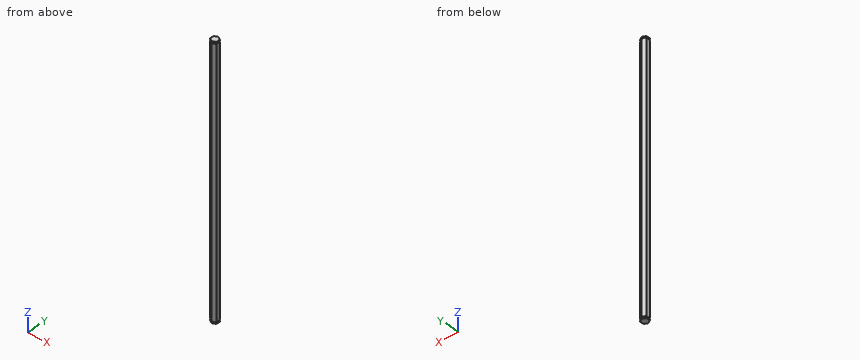
Solid Edge part; units mm, degrees
sketch "Sketch1" plane through (0, 0, 0) normal (0, 0, 1) x (1, 0, 0)
  line L0 (-6.1009, 4.0673) -> (-6.5728, -3.2499)
  line L1 (-6.5728, -3.2499) -> (-0.4719, -7.3171)
  line L2 (-0.4719, -7.3171) -> (6.1009, -4.0673)
  line L3 (6.1009, -4.0673) -> (6.5728, 3.2499)
  line L4 (6.5728, 3.2499) -> (0.4719, 7.3171)
  line L5 (0.4719, 7.3171) -> (-6.1009, 4.0673)
extrude "Protrusion1" add sketch "Sketch1" against normal blind 528.58
sketch "Sketch2" plane through (0, 0, -2) normal (0, 0, 1) x (-0.8964, -0.4432, 0)
  circle A0 centre (0, 0) radius 5.5
  circle A1 centre (0, 0) radius 13.1424
extrude "ExtrudedCutout_1" cut sketch "Sketch2" against normal blind 2
sketch "Sketch3" plane through (0, 0, -526.58) normal (0, 0, -1) x (0.8964, 0.4432, 0)
  circle A0 centre (0, 0) radius 5.5
  circle A1 centre (0, 0) radius 13.1424
extrude "ExtrudedCutout_2" cut sketch "Sketch3" against normal blind 2
properties part number "BumbleB0532"
Could you check a few things on this model? Use its own coordinates, in mm. Coordinates: 2 decimals unless noted, no trailing zeros. Order: outer loops, then holes, each group sorted by start corner. A loop starts at its lowest first (then second) coordinate and runs counter-clockwise, first axis right, second up.
Q1. Suppose I cut it at B-B on y = 0. Please give me the cut outline in (x, z).
Q2. Please list where these lines run through material, in increasing order: L1, parallel to X at y = 3.25, z = -429; L2, parallel to X at y = 3.5, z = -264; L3, parallel to Y at x = -1.75, z = -207.
Q3. Suppose I cut it at A-A on z = -156.5. Please give me the cut outline in (x, y), and give its area (3 significant figures).
Answer:
1. outline: (-6.36, -528.58) - (6.36, -528.58) - (6.36, -526.58) - (5.5, -526.58) - (5.5, -524.58) - (6.36, -524.58) - (6.36, -4) - (5.5, -4) - (5.5, -2) - (6.36, -2) - (6.36, 0) - (-6.36, 0) - (-6.36, -2) - (-5.5, -2) - (-5.5, -4) - (-6.36, -4) - (-6.36, -524.58) - (-5.5, -524.58) - (-5.5, -526.58) - (-6.36, -526.58) - close
2. L1: x = -6.15 to 6.57
2. L2: x = -6.14 to 6.2
2. L3: y = -6.47 to 6.22
3. outline: (-6.57, -3.25) - (-0.47, -7.32) - (6.1, -4.07) - (6.57, 3.25) - (0.47, 7.32) - (-6.1, 4.07) - close
3. area: 140 mm2
